Read the model definition and answer for the solid it produces. Units are mm, in the model's axes. A direction names the side the tool comes from. Coordinates: 2 decimals unless noted, no trailing zeros. Loops run counter-clockwise (first coordinate to the right, second up) from the corner with the lowest first, then second, coordinate; pieces in that order, holes last. Notation, with made-up numbers: (54, 14) -> (80, 14) arc R31 cw to (80, 52) -> close; hole circle Ø5 at (81.5, 53). An arc over 180 degrees is marked (long way). Answer as a JSON object with one key per item and string values. Group by question number.
Q1. For faces 4 (the cylindrical face through (-478.751, -230.885, -47.115)), 5 (the flat face through (-625, 29, -45)), 6 (the flat face through (-342, 280, 246)), 7 (the flat face through (342, -280, 246)), 8 (the flat face through (-3, -152, 500)), determine the directions among +Z, -Z, +X, -X, +Y, -Y from which every point of the face is accessible in a straight line to the end or side of a thin tool.
Q2. Straight lines are drawn through the part: line 1 along X through (y, z) = (-43.5, 470); line 2 along Y through (x, z) = (458.5, 134); line 3 along X through (y, z) = (-87, -30). For each, find the intervals that lie inside material, in ascending order. Write a range as [from, to].
Q3. Each of these flat-tipped pins is pushed along its axis until it touches: P1, Ø1, axis at x = 255.5, y = -234.5, coming from the +Z side; P2, Ø25, axis at x = -264.5, z = -44, coming from the -Y side; P3, Ø15, axis at y = 134, z = -45.5, coming from the -X side. Where does it stop, or does it pass through?
Q4. The part is cut by section C-C on y = 63.5. Write down the section's boundary in (x, z).
Q5. The part is cut by section A-A on z = 26. Write down the section's boundary in (x, y), and give its area (3 significant figures).
Q6. The part is cut by section B-B on x = 100. Write down the section's boundary in (y, z), and give its area (3 significant figures).
Q7. Determine the mould class of faces 1 (the flat face through (-3, -290, -20)), 2 (the flat face through (333, 255, 500)), 3 (the flat face through (-675, 4, 254)) for opening direction X: released by +X, released by -X, zero draft, split by the parting line, or undercut.
from build123d import *

# Parameters (mm, degrees)
F0_W     = 1350
F0_H     = 600
F0_W_2   = 20
F0_H_2   = 560
F1_DEPTH = 500
F2_W     = 1350
F2_H     = 70
F3_DEPTH = 20
F4_W     = 1350
F4_H     = 600
F5_DEPTH = 20
F6_R     = 25
F7_DEPTH = 55
F9_DEPTH = 50


with BuildPart() as f1:
    # F0 (on Top) → F1 (new body)
    with BuildSketch(Plane.XY):
        Rectangle(F0_W, F0_H)
        Polygon((-655, -280), (-655, 280), (-20, 280), (0, 280), (20, 280), (655, 280), (655, -280), (20, -280), (0, -280), (-20, -280), align=None, mode=Mode.SUBTRACT)
        with Locations((10, 0)):
            Rectangle(F0_W_2, F0_H_2)
        with Locations((-10, 0)):
            Rectangle(F0_W_2, F0_H_2)
    extrude(amount=F1_DEPTH)

    # F2 (on face) → F3 (join)
    with BuildSketch(Plane.XY.offset(500)):
        with Locations((0, 265)):
            Rectangle(F2_W, F2_H)
    extrude(amount=F3_DEPTH)

    # F4 (on face) → F5 (join)
    with BuildSketch(Plane(origin=(0, 0, 0), x_dir=(1, 0, 0), z_dir=(0, 0, -1))):
        Rectangle(F4_W, F4_H)
    extrude(amount=F5_DEPTH)

    # F6 (on face) → F7 (join)
    with BuildSketch(Plane(origin=(0, 0, -20), x_dir=(1, 0, 0), z_dir=(0, 0, -1))):
        with Locations((-502.596352, 223.376156)):
            Circle(F6_R)
        with Locations((-502.596352, -223.376156)):
            Circle(F6_R)
        with Locations((502.596352, -223.376156)):
            Circle(F6_R)
        with Locations((502.596352, 223.376156)):
            Circle(F6_R)
    extrude(amount=F7_DEPTH)

    # F8 (on face) → F9 (join)
    with BuildSketch(Plane(origin=(0, 0, -20), x_dir=(1, 0, 0), z_dir=(0, 0, -1))):
        Polygon((645, 270), (-645, 270), (-645, -270), (-645, -300), (-625, -300), (-625, -250), (-625, 250), (625, 250), (625, -250), (625, -300), (645, -300), (645, -270), align=None)
    extrude(amount=F9_DEPTH)


solid = f1.part
Final values:
{
 "1": {"face 4": "-Z", "face 5": "-Z, +Y", "face 6": "none", "face 7": "+Z", "face 8": "+Z, +X, -X, -Y"},
 "2": {"line 1": "x = [-675, -655], [-20, 20], [655, 675]", "line 2": "y = [-300, -280], [280, 300]", "line 3": "x = [-645, -625], [625, 645]"},
 "3": {"P1": "stops at z = 0", "P2": "stops at y = -270", "P3": "stops at x = -645"},
 "4": {"outline": "(-675, -20) -> (-645, -20) -> (-645, -70) -> (-625, -70) -> (-625, -20) -> (625, -20) -> (625, -70) -> (645, -70) -> (645, -20) -> (675, -20) -> (675, 500) -> (655, 500) -> (655, 0) -> (20, 0) -> (20, 500) -> (-20, 500) -> (-20, 0) -> (-655, 0) -> (-655, 500) -> (-675, 500) -> close"},
 "5": {"outline": "(-675, -300) -> (675, -300) -> (675, 300) -> (-675, 300) -> close; hole (-655, -280) -> (-20, -280) -> (-20, 280) -> (-655, 280) -> close; hole (20, -280) -> (655, -280) -> (655, 280) -> (20, 280) -> close", "area": "98,800 mm2"},
 "6": {"outline": "(-300, -20) -> (-270, -20) -> (-270, -70) -> (-250, -70) -> (-250, -20) -> (300, -20) -> (300, 520) -> (230, 520) -> (230, 500) -> (280, 500) -> (280, 0) -> (-280, 0) -> (-280, 500) -> (-300, 500) -> close", "area": "34,400 mm2"},
 "7": {"face 1": "zero draft", "face 2": "undercut", "face 3": "released by -X"}
}
